from build123d import *

# Parameters (mm, degrees)
SKETCH_R    = 1.5
SKETCH_R_2  = 1.25
PAD_DEPTH   = 3
FILLET_R    = 2
FILLET001_R = 1


with BuildPart() as part:
    # Sketch → Pad (new body)
    with BuildSketch(Plane.XY):
        Polygon((-5, -40.5), (-5, 3), (10, 3), (10, -10.5), (5, -15.5), (5, -40.5), align=None)
        Circle(SKETCH_R, mode=Mode.SUBTRACT)
        with Locations((5, 0)):
            Circle(SKETCH_R, mode=Mode.SUBTRACT)
        with Locations((0, -30)):
            Circle(SKETCH_R_2, mode=Mode.SUBTRACT)
    extrude(amount=PAD_DEPTH)

    # Fillet
    fillet_edges = [part.edges().sort_by_distance(p)[0] for p in [
        (10, 3, 1.5),
        (-5, 3, 1.5),
        (-5, -40.5, 1.5),
        (5, -40.5, 1.5),
    ]]
    fillet(fillet_edges, radius=FILLET_R)

    # Fillet001
    fillet001_edges = [part.edges().sort_by_distance(p)[0] for p in [
        (10, -10.5, 1.5),
        (5, -15.5, 1.5),
    ]]
    fillet(fillet001_edges, radius=FILLET001_R)


solid = part.part
Could you check a few things on this model? Use its own coordinates, in mm. A direction names the side the tool comes from. Give positions to 0.01 mm unless a question says otherwise; leave off trailing zeros. Write each loop counter-clockwise with the first axis right and the second up, starting at its lowest first coordinate (ties: lowest second). Pieces come first, ordered by that corner, then holes. Notation, with made-up numbers: (-35, -0.5) -> (18, -0.5) arc R12 cw to (18, 7.5) -> close; hole circle Ø1 at (-28, 48.5). An arc over 180 degrees is marked (long way). Write each question's results on one line, items separated by ' | '. Start each with the question number.
Q1. Suppose I cut it at A-A, the plane z = 0.95. List the corners of the cut face in (x, y) for me, and give its area (3 significant figures).
Q2. Suppose I cut it at B-B, the plane x = 0. List the corners of the cut face in (y, z) for me, and give its area (3 significant figures).
Q3. I'm going to push a flat-ended pin straight in: pin 1 Ø1.5 at (y, z) = (-25.5, 1.5) entering from +X. Where does the tip first touch, or does it pass through?
Q4. Suppose I cut it at C-C, the plane y = 0. List the corners of the cut face in (x, z) for me.
Q5. We'd pull the mould along Y, two halves only. Please class faces 3 (the face through (0.672, -28.946, 1.479)), 4 (the face through (-4.43, 2.4, 1.52)), 5 (the face through (1, -18, 0)): +Y half, -Y half, draft (parallel to the pull), parting line (faces both ways), or undercut.
Q6. I need wall thicknesses on probe 1 along Y at (x, z) = (0, 0.85); probe 2 along Y at (x, z) = (-0.5, 1.55); probe 3 along X at (y, z) = (-20, 1.85). Which ranges of each line are inside material? Lowest first, please.
Q7. Suppose I cut it at D-D, the plane y = -30. List the corners of the cut face in (x, z) for me.
Q8. Which directions (+Z, -Z, +X, -X, +Y, -Y) give clear straight access to the entire face, cutting with the end or side of a thin tool? Please do faces 1 (the face through (0, -40.5, 1)), 2 (the face through (5, -27, 1)).
Outcome:
1) outline: (-5, -38.5) arc R2 ccw to (-3, -40.5) -> (3, -40.5) arc R2 ccw to (5, -38.5) -> (5, -15.91) arc R1 cw to (5.29, -15.21) -> (9.71, -10.79) arc R1 ccw to (10, -10.09) -> (10, 1) arc R2 ccw to (8, 3) -> (-3, 3) arc R2 ccw to (-5, 1) -> close; hole circle Ø3 at (0, 0); hole circle Ø2.5 at (0, -30); hole circle Ø3 at (5, 0) | area: 493 mm2
2) outline: (-40.5, 0) -> (-31.25, 0) -> (-31.25, 3) -> (-40.5, 3) -> close; (-28.75, 0) -> (-1.5, 0) -> (-1.5, 3) -> (-28.75, 3) -> close; (1.5, 0) -> (3, 0) -> (3, 3) -> (1.5, 3) -> close | area: 114 mm2
3) pin 1: x = 5
4) outline: (-5, 0) -> (-1.5, 0) -> (-1.5, 3) -> (-5, 3) -> close; (1.5, 0) -> (3.5, 0) -> (3.5, 3) -> (1.5, 3) -> close; (6.5, 0) -> (10, 0) -> (10, 3) -> (6.5, 3) -> close
5) face 3: undercut | face 4: +Y half | face 5: draft
6) probe 1: -40.5 to -31.25, -28.75 to -1.5, 1.5 to 3 | probe 2: -40.5 to -31.15, -28.85 to -1.41, 1.41 to 3 | probe 3: -5 to 5
7) outline: (-5, 0) -> (-1.25, 0) -> (-1.25, 3) -> (-5, 3) -> close; (1.25, 0) -> (5, 0) -> (5, 3) -> (1.25, 3) -> close
8) face 1: +Z, -Z, +X, -X, -Y | face 2: +Z, -Z, +X, -Y
